Input: part model. Units: mm. Frame: model coordinates. Face numbers are marked on the shaded views. A direction names the side the tool comes from. Round coordinates to 2 decimals unless told otherwise and drop trailing zeros. Order: outer loops, then holes, each group sorted by start corner. A loop starts at its lowest first (then second) coordinate and runs counter-clockwise, first axis right, second up.
Item 1: First-contact query: pin 1 (1.5 mm diameter, centred on y = -39.5, z = -12, fed in from +X); pin 2 (11.5 mm diameter, centred on x = 23, z = 5, fed in from -Y); pin 3 (8.5 mm diameter, centred on y = 83, z = -6, fed in from +X). Flat tips, straight axial feed; report the tip coordinate or a pass-through.
Item 2: Cut plane A-A on z = 0. Output: boundary loops of the cut face in (x, y) (3 decimals), then the cut area to 3 significant figures.
Item 3: Reachability of the marked faces 1, 2 and 3 from +Z, -Z, +X, -X, +Y, -Y: full face, straight path, thin tool, end or side. Return the list, or none.
Item 4: Cut plane B-B on y = 68. Output: boundary loops of the cut face in (x, z) (3 decimals).
Item 5: Cut plane C-C on x = -7.5. Output: boundary loops of the cut face in (y, z).
Item 6: Cut plane D-D on z = -17.5. Output: boundary loops of the cut face in (x, y).
Item 7: Line query: L1, parallel to X at y = -72, z = 0.5; L2, parallel to Z at x = -13, y = -51.5; L3, parallel to X at y = 2.5, z = -10.5. Output: solid intervals per line, ascending.
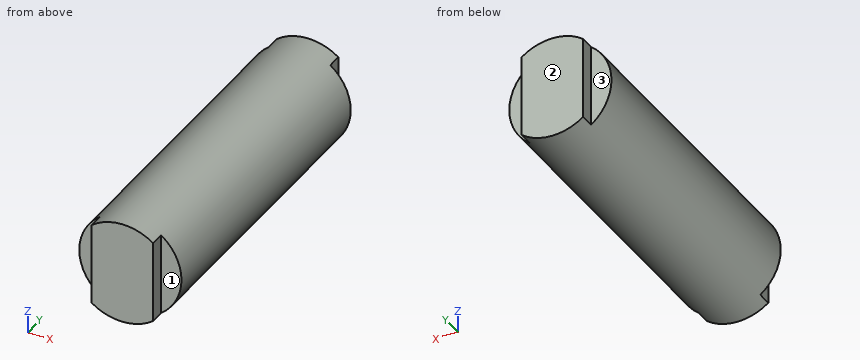
```python
from build123d import *

# Parameters (mm, degrees)
SKETCH2_R               = 26.415
EXTRUDE1_DEPTH          = 88.10625
SKETCH3_W               = 10.541
SKETCH3_H               = 7.62
EXTRUDE2_DEPTH          = 27.415
MIRROR2_COPY_1_SKETCH_W = 10.541
MIRROR2_COPY_1_SKETCH_H = 7.62
MIRROR2_COPY_1_DEPTH    = 27.415


with BuildPart() as part:
    # Sketch2 → Extrude1 (new body, symmetric)
    with BuildSketch(Plane(origin=(0, 0, 0), x_dir=(1, 0, 0), z_dir=(0, 1, 0))):
        Circle(SKETCH2_R)
    extrude(amount=EXTRUDE1_DEPTH, both=True)

    # Sketch3 → Extrude2 (cut, symmetric)
    with BuildSketch(Plane.XY):
        with Locations((21.1445, 84.29625)):
            Rectangle(SKETCH3_W, SKETCH3_H)
    extrude2 = extrude(amount=EXTRUDE2_DEPTH, both=True, mode=Mode.SUBTRACT)

    # Mirror1: Extrude2 across plane
    add(extrude2.mirror(Plane(origin=(0, 0, 0), x_dir=(0, 0, 1), z_dir=(1, 0, 0))), mode=Mode.SUBTRACT)

    # Mirror2: Extrude2 across plane
    add(extrude2.mirror(Plane.ZX), mode=Mode.SUBTRACT)

    # Mirror2 copy 1 sketch → Mirror2 copy 1 (cut, symmetric)
    with BuildSketch(Plane(origin=(0, 0, 0), x_dir=(-1, 0, 0), z_dir=(0, 0, 1))):
        with Locations((21.1445, 84.29625)):
            Rectangle(MIRROR2_COPY_1_SKETCH_W, MIRROR2_COPY_1_SKETCH_H)
    extrude(amount=MIRROR2_COPY_1_DEPTH, both=True, mode=Mode.SUBTRACT)


solid = part.part
```
From the geometry:
1. pin 1: stops at x = 23.9
1. pin 2: stops at y = -80.49
1. pin 3: stops at x = 26.29
2. outline: (-26.415, -80.486) - (-15.874, -80.486) - (-15.874, -88.106) - (15.874, -88.106) - (15.874, -80.486) - (26.415, -80.486) - (26.415, 80.486) - (15.874, 80.486) - (15.874, 88.106) - (-15.874, 88.106) - (-15.874, 80.486) - (-26.415, 80.486) - close
2. area: 8,990 mm2
3. face 1: +Z, -Z, +X, -Y
3. face 2: +Z, -Z, +X, -X, +Y
3. face 3: +Z, -Z, -X, +Y
4. outline: circle Ø52.83 at (0, 0)
5. outline: (-88.11, -25.33) - (88.11, -25.33) - (88.11, 25.33) - (-88.11, 25.33) - close
6. outline: (-19.79, -80.49) - (-15.87, -80.49) - (-15.87, -88.11) - (15.87, -88.11) - (15.87, -80.49) - (19.79, -80.49) - (19.79, 80.49) - (15.87, 80.49) - (15.87, 88.11) - (-15.87, 88.11) - (-15.87, 80.49) - (-19.79, 80.49) - close
7. L1: x = -26.41 to 26.41
7. L2: z = -22.99 to 22.99
7. L3: x = -24.24 to 24.24
